from build123d import *

# Parameters (mm, degrees)
SKETCH8_R               = 59.25
CUT_EXTRUDE4_DEPTH      = 5.5
CUT_EXTRUDE5_START      = -5.5
SKETCH9_R               = 59.25
CUT_EXTRUDE5_DEPTH      = 5.5
SKETCH11_R              = 43.435
BOSS_EXTRUDE1_DEPTH     = 6.5
CUT_EXTRUDE6_DEPTH      = 175.408285354
CUT_EXTRUDE6_DEPTH_BACK = 175.408285354
SKETCH12_R              = 19.84375
CUT_EXTRUDE7_DEPTH      = 175.408285354
CUT_EXTRUDE7_DEPTH_BACK = 175.408285354
SKETCH13_R              = 4.7625


# Read off the part's stored shape, not the designer's step: Shell3
with BuildPart() as part:
    # Sketch1 → Revolve1 (revolve)
    with BuildSketch(Plane.XY, mode=Mode.PRIVATE) as revolve1_sk:
        with BuildLine():
            Line((0, 209.55), (68, 209.55))
            Line((68, 209.55), (68, 204.4))
            Line((68, 204.4), (62.4, 204.4))
            Line((62.4, 204.4), (62.4, 192.9))
            Line((62.4, 192.9), (62.9, 192.9))
            Line((62.9, 192.9), (62.9, 188.6))
            ThreePointArc((62.9, 188.6), (62.755888959, 187.580323047), (62.334844366, 186.640519594))
            Line((62.334844366, 186.640519594), (47.372553847, 162.859973589))
            ThreePointArc((47.372553847, 162.859973589), (44.438305823, 156.31050954), (43.434, 149.204409302))
            Line((43.434, 149.204409302), (43.434, 64.204409302))
            ThreePointArc((43.434, 64.204409302), (45.964317306, 50.780645643), (53.207994273, 39.199234658))
            Line((53.207994273, 39.199234658), (60.495480053, 31.301573198))
            ThreePointArc((60.495480053, 31.301573198), (62.277511561, 28.452407038), (62.9, 25.15))
            Line((62.9, 25.15), (62.9, 16.65))
            Line((62.9, 16.65), (62.4, 16.65))
            Line((62.4, 16.65), (62.4, 5.15))
            Line((62.4, 5.15), (68, 5.15))
            Line((68, 5.15), (68, 0))
            Line((68, 0), (0, 0))
            Line((0, 0), (0, 209.55))
        make_face()
    revolve(revolve1_sk.sketch.rotate(Axis((0, 0, 0), (0, 1, 0)), 90), axis=Axis((0, 0, 0), (0, 1, 0)))

    # Shell3 outline → Shell3 (revolve, cut)
    with BuildSketch(Plane.XY):
        with BuildLine():
            Line((0, 208.55), (0, 1))
            Line((0, 1), (67, 1))
            Line((67, 1), (67, 4.15))
            Line((67, 4.15), (61.4, 4.15))
            Line((61.4, 4.15), (61.4, 17.65))
            Line((61.4, 17.65), (61.9, 17.65))
            Line((61.9, 17.65), (61.9, 25.15))
            ThreePointArc((61.9, 25.15), (61.346134368, 28.088351379), (59.7605531, 30.623426921))
            Line((59.7605531, 30.623426921), (52.47306732, 38.52108838))
            ThreePointArc((52.47306732, 38.52108838), (45.032940112, 50.416589983), (42.434, 64.204409302))
            Line((42.434, 64.204409302), (42.434, 149.204409302))
            ThreePointArc((42.434, 149.204409302), (43.477471904, 156.587634385), (46.526150206, 163.39251549))
            Line((46.526150206, 163.39251549), (61.488440725, 187.173061495))
            ThreePointArc((61.488440725, 187.173061495), (61.79505504, 187.857447892), (61.9, 188.6))
            Line((61.9, 188.6), (61.9, 191.9))
            Line((61.9, 191.9), (61.4, 191.9))
            Line((61.4, 191.9), (61.4, 205.4))
            Line((61.4, 205.4), (67, 205.4))
            Line((67, 205.4), (67, 208.55))
            Line((67, 208.55), (0, 208.55))
        make_face()
    revolve(axis=Axis((0, 0, 0), (0, 1, 0)), mode=Mode.SUBTRACT)

    # Sketch8 → Cut-Extrude4 (cut)
    with BuildSketch(Plane.XZ):
        with Locations(Location((0, 0, 0), (0, 0, 270))):
            Circle(SKETCH8_R)
    extrude(amount=-CUT_EXTRUDE4_DEPTH, mode=Mode.SUBTRACT)

    # Sketch9 → Cut-Extrude5 (cut)
    with BuildSketch(Plane(origin=(0, 209.55, 0), x_dir=(1, 0, 0), z_dir=(0, 1, 0)).offset(CUT_EXTRUDE5_START)):
        with Locations(Location((0, 0, 0), (0, 0, 90))):
            Circle(SKETCH9_R)
    extrude(amount=CUT_EXTRUDE5_DEPTH, mode=Mode.SUBTRACT)

    # Sketch11 → Boss-Extrude1 (add)
    with BuildSketch(Plane(origin=(0, 139, 0), x_dir=(1, 0, 0), z_dir=(0, 1, 0))):
        with Locations(Location((0, 0, 0), (0, 0, 90))):
            Circle(SKETCH11_R)
    extrude(amount=BOSS_EXTRUDE1_DEPTH)

    # Sketch12 → Cut-Extrude6 (cut, two sides: drawn at the far end of the back side and taken through both)
    with BuildSketch(Plane(origin=(0, 145.5, 0), x_dir=(1, 0, 0), z_dir=(0, 1, 0)).offset(-CUT_EXTRUDE6_DEPTH_BACK)):
        with Locations(Location((0, 0, 0), (0, 0, 270))):
            Circle(SKETCH12_R)
    extrude(amount=CUT_EXTRUDE6_DEPTH + CUT_EXTRUDE6_DEPTH_BACK, mode=Mode.SUBTRACT)

    # Sketch13 → Cut-Extrude7 (cut, two sides: drawn at the far end of the back side and taken through both)
    with BuildSketch(Plane(origin=(0, 145.5, 0), x_dir=(1, 0, 0), z_dir=(0, 1, 0)).offset(-CUT_EXTRUDE7_DEPTH_BACK)):
        with Locations(Location((0, 28.575, 0), (0, 0, 270))):
            Circle(SKETCH13_R)
        with Locations(Location((24.746675913, -14.2875, 0), (0, 0, 270))):
            Circle(SKETCH13_R)
        with Locations(Location((-24.746675913, -14.2875, 0), (0, 0, 270))):
            Circle(SKETCH13_R)
    extrude(amount=CUT_EXTRUDE7_DEPTH + CUT_EXTRUDE7_DEPTH_BACK, mode=Mode.SUBTRACT)


solid = part.part
Model file for the job. Use its own axes, mm. A direction names the side the tool comes from. Give positions to 0.01 mm unless a question says otherwise; leave off trailing zeros. Order: outer loops, then holes, each group sorted by start corner. A loop starts at its lowest first (then second) coordinate and runs counter-clockwise, first axis right, second up. Notation, with made-up numbers: (-23, -24.5) - (-9, -24.5) arc R26 ccw to (-9, 12.5) - close; hole circle Ø6 at (-9, 67.25). An arc over 180 degrees is marked (long way). One line per item, written item: value.
Item 1: Pin check, flat tips, straight feed: pin 1 Ø8 at (x, y) = (-52.5, 52.5) entering from -Z; pin 2 Ø2 at (x, z) = (-44, -19) entering from +Y; pin 3 Ø2 at (x, y) = (-32.5, 56.5) entering from -Z; pin 4 Ø1 at (x, z) = (37, 13.5) entering from -Y. Stop position of each tip, or through.
Response values:
pin 1: through
pin 2: y = 167.21
pin 3: z = -31.12
pin 4: y = 139
Item 2: Tool access for faces 1 (the cylindrical face through (5.961, 142.204, 18.927)), 2 (the cylindrical face through (-49.96, 209.04, -31.85)), 3 (the cylindrical face through (49.96, 0.49, -31.85)), 4 (the flat face through (4.65, 208.55, 59.24)): list every direction of +Z, -Z, +X, -X, +Y, -Y with a clear straight run to the whole face (end or side of a thin tool).
Response values:
face 1: +Y, -Y
face 2: +Y
face 3: -Y
face 4: none
Item 3: Wall check: line 1 (Y direction, x = 51.5, z = -41); line 2 (X direction, y = 23, z = 0); line 3 (X direction, y = 200.5, z = 0). Give the ranges that are in metal, low to high.
Response values:
line 1: 0 to 1, 4.15 to 5.15, 204.4 to 205.4, 208.55 to 209.55
line 2: -62.9 to -61.9, 61.9 to 62.9
line 3: -62.4 to -61.4, 61.4 to 62.4
Item 4: Two-plate mould, pull along Z, no slides. Class faces 5 (the cylindrical face through (-13.419, 21.452, 60.428)), 6 (the conical face through (52.4, 38.7, 11.6)), 7 (the flat face through (55, 5.15, 30)): released by +Z, released by -Z, zero draft, split by the parting line, or undercut.
Response values:
face 5: undercut
face 6: split by the parting line
face 7: zero draft
Item 5: Slice it at A-A (y = 103). List the corners of the cut face in (x, z), then the cut area to 3 significant figures.
Response values:
outline: circle Ø86.87 at (0, 0); hole circle Ø84.87 at (0, 0)
area: 270 mm2
